from build123d import *

# Parameters (mm, degrees)
BOSS_EXTRUDE1_DEPTH = 20
FILLET1_R           = 2
SKETCH2_R           = 1.9
SKETCH2_R_2         = 2.2
CUT_EXTRUDE1_DEPTH  = 40


with BuildPart() as part:
    # Sketch1 → Boss-Extrude1 (new body)
    with BuildSketch(Plane.XY):
        Polygon((-25.4, 0), (25.4, 0), (25.4, 50), (28.9, 50), (28.9, -3), (7.3, -3), (7.3, -23), (4.3, -23), (4.3, -3), (-16.3, -3), (-16.3, -23), (-19.3, -23), (-19.3, -3), (-28.4, -3), (-28.4, 110.5), (-25.4, 110.5), align=None)
    extrude(amount=BOSS_EXTRUDE1_DEPTH)

    # Fillet1
    fillet1_edges = [part.edges().sort_by_distance(p)[0] for p in [
        (27.15, 50, 0),
        (5.8, -23, 0),
        (-17.8, -23, 0),
        (-17.8, -23, 20),
        (-26.9, 110.5, 0),
        (-25.4, 0, 10),
        (28.9, -3, 10),
        (7.3, -3, 10),
        (-19.3, -3, 10),
        (-28.4, -3, 10),
        (5.8, -23, 20),
        (27.15, 50, 20),
        (-26.9, 110.5, 20),
    ]]
    fillet(fillet1_edges, radius=FILLET1_R)

    # Sketch2 → Cut-Extrude1 (cut)
    with BuildSketch(Plane.ZY.offset(28.4)):
        with Locations(Location((10, 99.5, 0), (0, 0, 270))):
            Circle(SKETCH2_R)
        with Locations(Location((10, 15.5, 0), (0, 0, 270))):
            Circle(SKETCH2_R)
        with Locations(Location((10, -13, 0), (0, 0, 270))):
            Circle(SKETCH2_R_2)
    extrude(amount=-CUT_EXTRUDE1_DEPTH, mode=Mode.SUBTRACT)


solid = part.part
Work out the finished part from the listing and answer in its coordinate system (mm). A direction names the side the tool comes from. Give positions to 0.01 mm unless a question says otherwise; leave off trailing zeros. Loops run counter-clockwise (first coordinate to the right, second up) from the corner with the lowest first, then second, coordinate; pieces in that order, holes last. Notation, with made-up numbers: (-22, 63) -> (33, 63) arc R37 ccw to (33, 100) -> close; hole circle Ø10 at (5.25, 88.5). An arc over 180 degrees is marked (long way). Use a Markdown table: item, result. Add a question column.
1. Section D-D on y = 15.5 is taken. Determine the outline of the cut face in (x, z), and give its area (3 significant figures).
2. Find the intervals of material crossed by probe 1 along Z at (x, y) = (-26.15, 99.5); probe 2 along X at (y, z) = (-7.5, 4.25); probe 3 along Z at (x, y) = (-18, -13), in increasing order.
3. Determine the mould class of faces 1 (the flat face through (27, 50, 10)), 2 (the cylindrical face through (5.78, -15.1, 10.66)), 3 (the flat face through (-27, 25, 20)), 4 (the cylindrical face through (-26.92, 101.4, 10.08)) for opening direction Y: released by +Y, released by -Y, zero draft, split by the parting line, or undercut.
4. Section A-A on y = -13 is taken. Determine the outline of the cut face in (x, z), and give its area (3 significant figures).
5. Section C-C on x = -18 is taken. Determine the outline of the cut face in (y, z).
6. For faces 5 (the flat face through (18, -3, 10)), 6 (the flat face through (-19.3, -16, 10)), 7 (the flat face through (-25.4, 57, 10)), determine the directions among +Z, -Z, +X, -X, +Y, -Y from which every point of the face is accessible in a straight line to the end or side of a thin tool.
7. Flat-ended cylindrical pins translate along their axes: pin 1 Ø3 at (x, z) = (15, 10.5) entering from -Y; pin 2 Ø9 at (y, z) = (-13, 9.5) entering from +X; pin 3 Ø6 at (y, z) = (99.5, 10) entering from +X. Find the tip coordinate at first contact, or state that the pin passes through.
8. Section B-B on y = 99.5 is taken. Determine the outline of the cut face in (x, z).
Results below:
| question | item | result |
|---|---|---|
| 1 | outline | (-28.4, 0) -> (-25.4, 0) -> (-25.4, 8.1) -> (-28.4, 8.1) -> close; (-28.4, 11.9) -> (-25.4, 11.9) -> (-25.4, 20) -> (-28.4, 20) -> close; (25.4, 0) -> (28.9, 0) -> (28.9, 20) -> (25.4, 20) -> close |
| 1 | area | 119 mm^2 |
| 2 | probe 1 | z = 0 to 8.1, 11.9 to 20 |
| 2 | probe 2 | x = -19.3 to -16.3, 4.3 to 7.3 |
| 2 | probe 3 | z = 0 to 7.8, 12.2 to 20 |
| 3 | face 1 | released by +Y |
| 3 | face 2 | undercut |
| 3 | face 3 | zero draft |
| 3 | face 4 | undercut |
| 4 | outline | (-19.3, 0) -> (-16.3, 0) -> (-16.3, 7.8) -> (-19.3, 7.8) -> close; (-19.3, 12.2) -> (-16.3, 12.2) -> (-16.3, 20) -> (-19.3, 20) -> close; (4.3, 0) -> (7.3, 0) -> (7.3, 7.8) -> (4.3, 7.8) -> close; (4.3, 12.2) -> (7.3, 12.2) -> (7.3, 20) -> (4.3, 20) -> close |
| 4 | area | 93.6 mm^2 |
| 5 | outline | (-23, 2) arc R2 ccw to (-21, 0) -> (0, 0) -> (0, 20) -> (-21, 20) arc R2 ccw to (-23, 18) -> close; hole circle Ø4.4 at (-13, 10) |
| 6 | face 5 | +Z, -Z, +X, -Y |
| 6 | face 6 | +Z, -Z, -X, -Y |
| 6 | face 7 | +Z, -Z, +Y |
| 7 | pin 1 | stops at y = -3 |
| 7 | pin 2 | stops at x = 7.3 |
| 7 | pin 3 | stops at x = -25.4 |
| 8 | outline | (-28.4, 0) -> (-25.4, 0) -> (-25.4, 8.1) -> (-28.4, 8.1) -> close; (-28.4, 11.9) -> (-25.4, 11.9) -> (-25.4, 20) -> (-28.4, 20) -> close |
